Input: part model. Units: mm. Frame: model coordinates. Face numbers are marked on the shaded views. Give positions to 0.01 mm unless a question says otherwise; leave off trailing zeros. Answer as a JSON object with one key per item and string values.
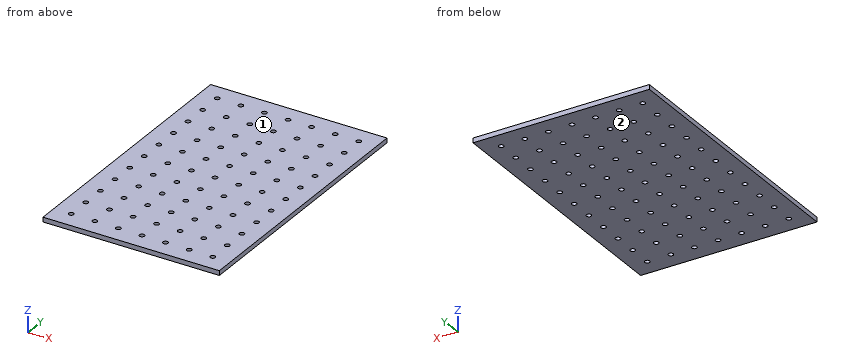
from build123d import *

# Parameters (mm, degrees)
F0_W     = 718
F0_H     = 1102
F1_DEPTH = 19.05
F2_R     = 10
F3_DEPTH = 19.051


with BuildPart() as f1:
    # F0 (on Top) → F1 (new body)
    with BuildSketch(Plane.XY):
        with Locations((359, -551)):
            Rectangle(F0_W, F0_H)
    extrude(amount=-F1_DEPTH)

    # F2 (on face) → F3 (cut, through all)
    with BuildSketch(Plane(origin=(0, 0, -19.05), x_dir=(1, 0, 0), z_dir=(0, 0, -1))):
        with Locations((359, 551)):
            Circle(F2_R)
        with Locations((263, 551)):
            Circle(F2_R)
        with Locations((647, 935)):
            Circle(F2_R)
        with Locations((263, 935)):
            Circle(F2_R)
        with Locations((359, 263)):
            Circle(F2_R)
        with Locations((71, 263)):
            Circle(F2_R)
        with Locations((551, 1031)):
            Circle(F2_R)
        with Locations((647, 167)):
            Circle(F2_R)
        with Locations((263, 743)):
            Circle(F2_R)
        with Locations((71, 71)):
            Circle(F2_R)
        with Locations((455, 359)):
            Circle(F2_R)
        with Locations((647, 263)):
            Circle(F2_R)
        with Locations((263, 839)):
            Circle(F2_R)
        with Locations((359, 71)):
            Circle(F2_R)
        with Locations((71, 359)):
            Circle(F2_R)
        with Locations((263, 167)):
            Circle(F2_R)
        with Locations((647, 455)):
            Circle(F2_R)
        with Locations((455, 71)):
            Circle(F2_R)
        with Locations((455, 1031)):
            Circle(F2_R)
        with Locations((455, 167)):
            Circle(F2_R)
        with Locations((359, 359)):
            Circle(F2_R)
        with Locations((167, 263)):
            Circle(F2_R)
        with Locations((167, 359)):
            Circle(F2_R)
        with Locations((71, 647)):
            Circle(F2_R)
        with Locations((359, 455)):
            Circle(F2_R)
        with Locations((551, 839)):
            Circle(F2_R)
        with Locations((455, 263)):
            Circle(F2_R)
        with Locations((647, 839)):
            Circle(F2_R)
        with Locations((167, 935)):
            Circle(F2_R)
        with Locations((263, 1031)):
            Circle(F2_R)
        with Locations((167, 455)):
            Circle(F2_R)
        with Locations((551, 647)):
            Circle(F2_R)
        with Locations((263, 359)):
            Circle(F2_R)
        with Locations((167, 551)):
            Circle(F2_R)
        with Locations((551, 743)):
            Circle(F2_R)
        with Locations((647, 551)):
            Circle(F2_R)
        with Locations((359, 1031)):
            Circle(F2_R)
        with Locations((71, 743)):
            Circle(F2_R)
        with Locations((71, 551)):
            Circle(F2_R)
        with Locations((647, 743)):
            Circle(F2_R)
        with Locations((71, 839)):
            Circle(F2_R)
        with Locations((551, 71)):
            Circle(F2_R)
        with Locations((647, 71)):
            Circle(F2_R)
        with Locations((359, 167)):
            Circle(F2_R)
        with Locations((167, 167)):
            Circle(F2_R)
        with Locations((167, 647)):
            Circle(F2_R)
        with Locations((167, 839)):
            Circle(F2_R)
        with Locations((71, 167)):
            Circle(F2_R)
        with Locations((647, 359)):
            Circle(F2_R)
        with Locations((263, 71)):
            Circle(F2_R)
        with Locations((647, 1031)):
            Circle(F2_R)
        with Locations((263, 647)):
            Circle(F2_R)
        with Locations((263, 455)):
            Circle(F2_R)
        with Locations((551, 455)):
            Circle(F2_R)
        with Locations((551, 359)):
            Circle(F2_R)
        with Locations((71, 935)):
            Circle(F2_R)
        with Locations((71, 455)):
            Circle(F2_R)
        with Locations((455, 935)):
            Circle(F2_R)
        with Locations((551, 935)):
            Circle(F2_R)
        with Locations((551, 263)):
            Circle(F2_R)
        with Locations((71, 1031)):
            Circle(F2_R)
        with Locations((359, 935)):
            Circle(F2_R)
        with Locations((455, 839)):
            Circle(F2_R)
        with Locations((551, 551)):
            Circle(F2_R)
        with Locations((359, 647)):
            Circle(F2_R)
        with Locations((455, 743)):
            Circle(F2_R)
        with Locations((455, 647)):
            Circle(F2_R)
        with Locations((455, 551)):
            Circle(F2_R)
        with Locations((359, 839)):
            Circle(F2_R)
        with Locations((167, 1031)):
            Circle(F2_R)
        with Locations((647, 647)):
            Circle(F2_R)
        with Locations((359, 743)):
            Circle(F2_R)
        with Locations((167, 743)):
            Circle(F2_R)
        with Locations((167, 71)):
            Circle(F2_R)
        with Locations((551, 167)):
            Circle(F2_R)
        with Locations((263, 263)):
            Circle(F2_R)
        with Locations((455, 455)):
            Circle(F2_R)
    extrude(amount=-F3_DEPTH, mode=Mode.SUBTRACT)


solid = f1.part
Item 1: Contact query for flat-ended pins moving along their axis: P1, Ø10, axis at x = 138.5, z = -9.5, coming from the +Y side; P2, Ø16, axis at x = 551, y = -167, coming from the -Z side. Output: stop coordinate, or through.
Geometry check:
{"P1": "stops at y = 0", "P2": "passes through"}
Item 2: Mould query, pull axis Z, two halves, no side actions, for the marked faces 1 and 2. Classes: released by +Z, released by -Z, zero draft, split by the parting line, or undercut.
Geometry check:
{"face 1": "released by +Z", "face 2": "released by -Z"}
Item 3: Cut plane A-A (z = -13). Give the number of separate pieces and of enclosed holes in the cut face, then the cut area to 3 significant figures.
Geometry check:
{"separate pieces": "1", "enclosed holes": "77", "area": "767,000 mm2"}
